from build123d import *

# Parameters (mm, degrees)
F0_W     = 180
F0_H     = 117
F2_DEPTH = 7
F1_W     = 170
F1_H     = 107
F3_DEPTH = 25
F4_R     = 3
F5_R     = 1
F6_R     = 1


with BuildPart() as f2:
    # F0 (on Top) → F2 (new body)
    with BuildSketch(Plane.XY):
        with Locations((-29.744874835, 27.1624445021)):
            Rectangle(F0_W, F0_H)
    extrude(amount=F2_DEPTH)

    # F1 (on face) → F3 (cut)
    with BuildSketch(Plane.XY):
        with Locations((-29.744874835, 27.1624445021)):
            Rectangle(F1_W, F1_H)
    extrude(amount=F3_DEPTH, mode=Mode.SUBTRACT)

    # F4
    f4_edges = [f2.edges().sort_by_distance(p)[0] for p in [
        (60.255125, 85.662445, 3.5),
        (60.255125, -31.337555, 3.5),
        (-119.744875, -31.337555, 3.5),
        (-119.744875, 85.662445, 3.5),
    ]]
    fillet(f4_edges, radius=F4_R)

    # F5
    f5_edges = [f2.edges().sort_by_distance(p)[0] for p in [
        (-119.744875, 27.162445, 7),
        (-29.744875, -31.337555, 7),
        (-118.866195, -30.458876, 7),
    ]]
    fillet(f5_edges, radius=F5_R)

    # F6
    f6_edges = [f2.edges().sort_by_distance(p)[0] for p in [
        (55.255125, -26.337555, 3.5),
        (55.255125, 80.662445, 3.5),
        (-114.744875, 80.662445, 3.5),
        (-114.744875, -26.337555, 3.5),
    ]]
    fillet(f6_edges, radius=F6_R)


solid = f2.part
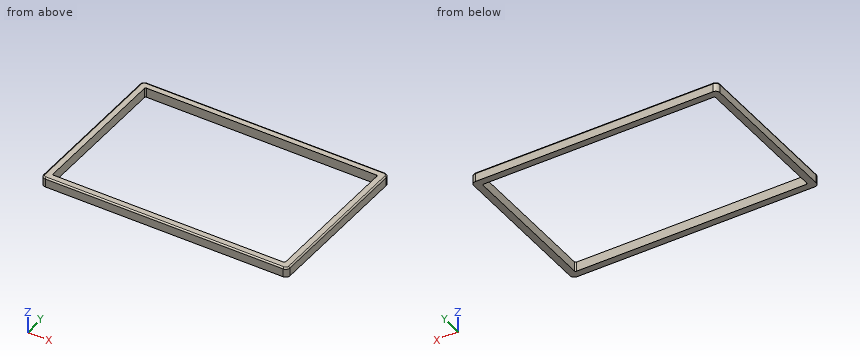
Geometry check sheet. Reference: the model listing, model coordinates, mm. Round coordinates to 2 decimals unless told otherwise and drop trailing zeros. Loops run counter-clockwise (first coordinate to the right, second up) from the corner with the lowest first, then second, coordinate; pieces in that order, holes last. Notation, with made-up numbers: (60.5, -34.75) - (105.5, -34.75) arc R17 cw to (105.5, -5.75) - close; hole circle Ø6 at (6, 43.5). An arc over 180 degrees is marked (long way). One line per question, with ' | ' between items. Start each with the question number.
1. Cross-section at B-B on y = 45. Record the cut outline in (x, z), then the cut area to 3 significant figures.
2. Cross-section at C-C on z = 3. Record the cut outline in (x, y), then the cut area to 3 significant figures.
3. Scan lines: line 1 (X direction, y = 25, z = 5.25); line 2 (Y direction, x = 4, z = 4); line 3 (X direction, y = 10, z = 6.25). Record each from-to range of solid material in increasing order. Write a range as [from, to].
4. Cross-section at A-A on x = -87.5. Record the cut outline in (y, z), then the cut area to 3 significant figures.
Taken from the geometry:
1) outline: (-119.74, 0) - (-114.74, 0) - (-114.74, 7) - (-118.74, 7) arc R1 ccw to (-119.74, 6) - close; (55.26, 0) - (60.26, 0) - (60.26, 6) arc R1 ccw to (59.26, 7) - (55.26, 7) - close | area: 69.6 mm²
2) outline: (-119.74, -28.34) arc R3 ccw to (-116.74, -31.34) - (57.26, -31.34) arc R3 ccw to (60.26, -28.34) - (60.26, 82.66) arc R3 ccw to (57.26, 85.66) - (-116.74, 85.66) arc R3 ccw to (-119.74, 82.66) - close; hole (-114.74, -25.34) arc R1 ccw to (-113.74, -26.34) - (54.26, -26.34) arc R1 ccw to (55.26, -25.34) - (55.26, 79.66) arc R1 ccw to (54.26, 80.66) - (-113.74, 80.66) arc R1 ccw to (-114.74, 79.66) - close | area: 2,860 mm²
3) line 1: [-119.74, -114.74], [55.26, 60.26] | line 2: [-31.34, -26.34], [80.66, 85.66] | line 3: [-119.71, -114.74], [55.26, 60.22]
4) outline: (-31.34, 0) - (-26.34, 0) - (-26.34, 7) - (-30.34, 7) arc R1 ccw to (-31.34, 6) - close; (80.66, 0) - (85.66, 0) - (85.66, 6) arc R1 ccw to (84.66, 7) - (80.66, 7) - close | area: 69.6 mm²
